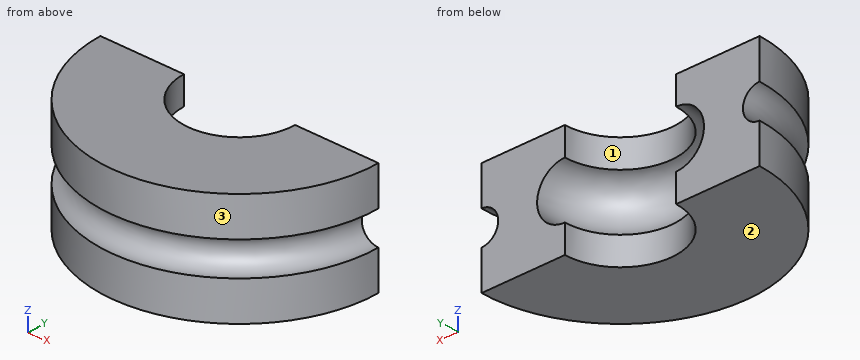
```python
from build123d import *

# Parameters (mm, degrees)
REVOLUTION_ANGLE = -180
SKETCH001_R      = 6
GROOVE_ANGLE     = 180


with BuildPart() as part:
    # Sketch → Revolution (revolve)
    with BuildSketch(Plane.XZ):
        with BuildLine():
            Line((20, 40), (50, 40))
            Line((50, 40), (50, 0))
            Line((50, 0), (20, 0))
            Line((20, 0), (20, 10))
            ThreePointArc((20, 10), (30, 20), (20, 30))
            Line((20, 30), (20, 40))
        make_face()
    revolve(axis=Axis((0, 0, 0), (0, 0, 1)), revolution_arc=REVOLUTION_ANGLE)

    # Sketch001 (on Face8 of Revolution) → Groove (revolve, cut)
    with BuildSketch(Plane(origin=(0, 0, 0), x_dir=(1, 0, 0), z_dir=(0, 1, 0))):
        with Locations((50, -20)):
            Circle(SKETCH001_R)
    revolve(axis=Axis((0, 0, 0), (0, 0, -1)), revolution_arc=GROOVE_ANGLE, mode=Mode.SUBTRACT)


solid = part.part
```
Geometry check sheet. Reference: the model listing, model coordinates, mm. Face numbers are marked on the shaded views. Give positions to 0.01 mm unless a question says otherwise; leave off trailing zeros. Write each loop counter-clockwise with the first axis right and the second up, starting at its lowest first coordinate (ties: lowest second). Pieces come first, ordered by that corner, then holes.
1) Gauge pin test, flat ends, axial feed: pin 1 (8 mm diameter, centred on y = -8.5, z = 5, fed in from +X); pin 2 (6 mm diameter, centred on y = -42.5, z = 13, fed in from -X); pin 3 (2 mm diameter, centred on y = -25, z = 16.5, fed in from +X). Record the tip position at first contact, or that the pin passes through.
2) Material ranges on L1, parallel to X at y = -10, z = 22; L2, parallel to Z at x = 11, y = -27; L3, parallel to X at y = -14, z = 36, recorded low to high.
3) Section check A-A, the plane x = 0. Record the boundary of the cut face in (y, z), and give its area (3 significant figures).
4) Section check C-C, the plane z = 11.5. Record the boundary of the cut face in (x, y).
5) Release check for a two-part mould opening along X. For the marked faces 1, 2 and 3 record: pulls with the +X half, pulls with the -X half, needs draft (parallel to the pull), parting line crosses it, or undercut.
6) Section check B-B, the plane z = 36.5. Record the boundary of the cut face in (x, y).
Computed:
1. pin 1: stops at x = 49.8
1. pin 2: stops at x = -30.66
1. pin 3: stops at x = 38.8
2. L1: x = -43.2 to -28.07, 28.07 to 43.2
2. L2: z = 0 to 15.98, 24.02 to 40
2. L3: x = -48 to -14.28, 14.28 to 48
3. outline: (-50, 0) - (-20, 0) - (-20, 10) arc R10 cw to (-20, 30) - (-20, 40) - (-50, 40) - (-50, 26) arc R6 cw to (-50, 14) - close
3. area: 986 mm2
4. outline: (-50, 0) arc R50 ccw to (50, 0) - (25.27, 0) arc R25.27 cw to (-25.27, 0) - close
5. face 1: undercut
5. face 2: needs draft
5. face 3: parting line crosses it
6. outline: (-50, 0) arc R50 ccw to (50, 0) - (20, 0) arc R20 cw to (-20, 0) - close
